from build123d import *

# Parameters (mm, degrees)
F0_W     = 2.8
F0_H     = 8
F1_DEPTH = 43
F2_R     = 3.99999
F3_R     = 1.5
F4_DEPTH = 5
F5_R     = 0.5


# Not quite as in the source:
# - a fillet or chamfer is up to 0.001 mm smaller than in the source, because OpenCascade refuses the exact size


with BuildPart() as f1:
    # F0 (on Top) → F1 (new body)
    with BuildSketch(Plane.XY):
        Rectangle(F0_W, F0_H)
    extrude(amount=F1_DEPTH)

    # F2 (radius 4 in the source; OpenCascade refuses exactly that, so slightly less here)
    f2_edges = [f1.edges().sort_by_distance(p)[0] for p in [
        (0, 4, 0),
        (0, -4, 0),
        (0, -4, 43),
        (0, 4, 43),
    ]]
    fillet(f2_edges, radius=F2_R)

    # F3 (on face) → F4 (cut)
    with BuildSketch(Plane(origin=(-1.4, 0, 0), x_dir=(0, -1, 0), z_dir=(-1, 0, 0))):
        with Locations((0, 4)):
            Circle(F3_R)
        with Locations((0, 39)):
            Circle(F3_R)
    extrude(amount=-F4_DEPTH, mode=Mode.SUBTRACT)

    # F5
    f5_edges = [f1.edges().sort_by_distance(p)[0] for p in [
        (-1.4, 4, 21.5),
        (1.4, 4, 21.5),
    ]]
    fillet(f5_edges, radius=F5_R)


solid = f1.part
Geometry check sheet. Reference: the model listing, model coordinates, mm. Give positions to 0.01 mm unless a question says otherwise; leave off trailing zeros. Use a Markdown table: item, result.
Item 1: Draft check along Y on faces 1 (the cylindrical face through (-0.02, 0.325, 37.536)), 2 (the cylindrical face through (0.013, 2.859, 1.203)), 3 (the flat face through (1.4, 0, 21)). Enter one of: +Y half, -Y half, draft (parallel to the pull), parting line (faces both ways), or undercut.
Answers follow:
| item | result |
|---|---|
| face 1 | undercut |
| face 2 | +Y half |
| face 3 | draft |
Item 2: Section check A-A (x = 0.45). State how many separate pieces and enclosed holes the cut face has, and give its area (3 significant figures).
Answers follow:
| item | result |
|---|---|
| separate pieces | 1 |
| enclosed holes | 2 |
| area | 316 mm2 |
Item 3: Material ranges on line 1 along Z through (x, y) = (0.7, 0); line 2 along Z through (x, y) = (0.7, 1); line 3 along Y through (x, z) = (0.3, 40), recorded low to high.
Answers follow:
| item | result |
|---|---|
| line 1 | z = 0 to 2.5, 5.5 to 37.5, 40.5 to 43 |
| line 2 | z = 0.13 to 2.88, 5.12 to 37.88, 40.12 to 42.87 |
| line 3 | y = -3.87 to -1.12, 1.12 to 3.87 |
